```python
from build123d import *

# Parameters (mm, degrees)
F1_DEPTH = 63.5
F0_W     = 25.4
F0_H     = 19.05
F2_DEPTH = 25.4
F3_DEPTH = 7.9375
F5_R     = 6.35
F6_SIZE  = 3.81


with BuildPart() as f1:
    # F0 (on Front) → F1 (new body, symmetric)
    with BuildSketch(Plane.XZ):
        Polygon((-41.275, -9.525), (41.275, -9.525), (41.275, 9.525), (22.225, 9.525), (-41.275, 9.525), align=None)
    extrude(amount=F1_DEPTH, both=True)

    # F0 (on Front) → F2 (join, symmetric)
    with BuildSketch(Plane.XZ):
        with BuildLine():
            Line((22.225, 9.525), (41.275, 9.525))
            Line((41.275, 9.525), (41.275, 27.0002))
            ThreePointArc((41.275, 27.0002), (45.9246798487, 38.2255201513), (57.15, 42.8752))
            Line((57.15, 42.8752), (60.325, 42.8752))
            Line((60.325, 42.8752), (60.325, 61.9252))
            Line((60.325, 61.9252), (57.15, 61.9252))
            ThreePointArc((57.15, 61.9252), (32.4542956671, 51.6959043329), (22.225, 27.0002))
            Line((22.225, 27.0002), (22.225, 9.525))
        make_face()
        with Locations((73.025, 52.4002)):
            Rectangle(F0_W, F0_H)
    extrude(amount=F2_DEPTH, both=True)

    # F0 (on Front) → F3 (join, symmetric)
    with BuildSketch(Plane.XZ):
        with BuildLine():
            add(Edge.make_bspline(
                [(-41.275, 9.525), (-40.3791815042, 47.0926873386), (9.2821996659, 61.9340203702), (57.15, 61.9252)],
                knots=[0, 0, 0, 0, 111.5045361635, 111.5045361635, 111.5045361635, 111.5045361635], degree=3))
            Line((-41.275, 9.525), (22.225, 9.525))
            Line((22.225, 9.525), (22.225, 27.0002))
            ThreePointArc((22.225, 27.0002), (32.4542956671, 51.6959043329), (57.15, 61.9252))
        make_face()
    extrude(amount=F3_DEPTH, both=True)

    # F0 (on Front) → F4 (revolve)
    with BuildSketch(Plane.XZ):
        Polygon((85.725, 66.675), (85.725, 61.9252), (85.725, 42.8752), (85.725, 38.1), (111.125, 38.1), (111.125, 66.675), align=None)
    revolve(axis=Axis((85.725, 0, 52.3875), (0, 0, -1)))

    # F5
    f5_edges = [f1.edges().sort_by_distance(p)[0] for p in [
        (41.275, 63.5, 0),
        (-41.275, 63.5, 0),
        (41.275, -63.5, 0),
        (-41.275, -63.5, 0),
    ]]
    fillet(f5_edges, radius=F5_R)

    # F6
    f6_edges = [f1.edges().sort_by_distance(p)[0] for p in [
        (60.325, 0, 66.675),
        (60.325, 0, 38.1),
    ]]
    chamfer(f6_edges, length=F6_SIZE)


solid = f1.part
```
Design review of the part built by this model. Coordinates are the model's own, in mm. A direction names the side the tool comes from. Give positions to 0.01 mm unless a question says otherwise; leave off trailing zeros. Write each loop counter-clockwise with the first axis right and the second up, starting at its lowest first coordinate (ties: lowest second). Pieces come first, ordered by that corner, then holes. Notation, with made-up numbers: (-37.5, 3) - (-8.5, 3) arc R19 cw to (-8.5, 23) - close; hole circle Ø10 at (73.5, -21.75). An arc over 180 degrees is marked (long way). Return JSON: item names as keys, results as strings. Group by question number.
(1) Insertion check: pin 1 (10 mm diameter, centred on y = -7, z = 47.5, fed in from +X); pin 2 (4 mm diameter, centred on x = -5.5, z = 32.5, fed in from +Y); pin 3 (11 mm diameter, centred on y = 17, z = 11.5, fed in from +X) (3 decimals). Each pin has a flat end and moves straight along its axis. Give the tip position at first contact, or say it passes through.
(2) We need section A-A, the plane z = -0.5. Give the boundary of the cut face in (x, y) (3 decimals), then the cut area to 3 significant figures.
(3) Machinability: for faces 1 (the flat face through (60, -2, 61.925)), 2 (the flat face through (-2, 7.938, 30)), 3 (the flat face through (22.225, -17, 18)), 4 (the flat face through (46, 25.4, 42)), which of the approach directions +Z, -Z, +X, -X, +Y, -Y give a long, thin tool a straight path to every point of the face, cutting with its end or side? Answer none if there is none.
(4) We need section B-B, the plane y = -44. Give the boundary of the cut face in (x, z) (3 decimals), then the cut area to 3 significant figures.
(5) To check wall thickness, follow probe 1 along Z at (x, y) = (1, 28) (3 decimals); probe 2 along X at (y, z) = (31.5, 6) (3 decimals); probe 3 along Z at (x, y) = (75, 0.5) (3 decimals). State the ranges of each line that lie inside material, in increasing order.
(6) Mouldability with a two-part tool opening along X and no side actions: class faces 5 (the cylindrical face through (45.8, -0.4, 38.1)), 6 (the conical face through (68.445, 13.25, 66.49)), 7 (the flat face through (1, -36, 9.525)), 8 (the flat face through (22.225, 17, 18)) as +X half, -X half, draft (parallel to the pull), parting line (faces both ways), or undercut.
Reported:
{
 "1": {"pin 1": "stops at x = 111.05", "pin 2": "stops at y = 7.94", "pin 3": "stops at x = 41.275"},
 "2": {"outline": "(-41.275, -57.15) arc R6.35 ccw to (-34.925, -63.5) - (34.925, -63.5) arc R6.35 ccw to (41.275, -57.15) - (41.275, 57.15) arc R6.35 ccw to (34.925, 63.5) - (-34.925, 63.5) arc R6.35 ccw to (-41.275, 57.15) - close", "area": "10,400 mm2"},
 "3": {"face 1": "+Z, -X", "face 2": "+Z, -X, +Y", "face 3": "+Z, -X, -Y", "face 4": "+Z, +X, -X, +Y"},
 "4": {"outline": "(-41.275, -9.525) - (41.275, -9.525) - (41.275, 9.525) - (-41.275, 9.525) - close", "area": "1,570 mm2"},
 "5": {"probe 1": "z = -9.525 to 9.525", "probe 2": "x = -41.275 to 41.275", "probe 3": "z = 38.1 to 66.675"},
 "6": {"face 5": "undercut", "face 6": "parting line", "face 7": "draft", "face 8": "-X half"}
}
